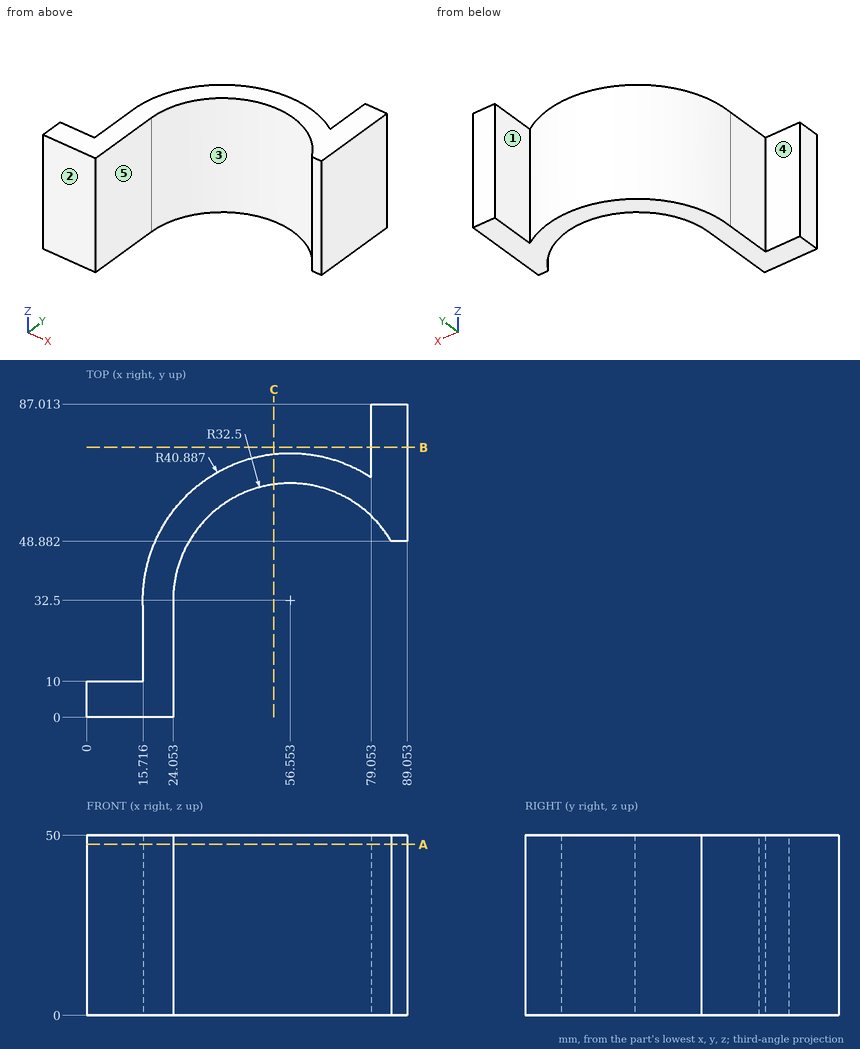
Can you work these out from the drawing? Everything is in mm from the part's minimum corner. A direction names the side the tool comes from. Coordinates: 2 decimals unless noted, no trailing zeros. Loops run counter-clockwise (first coordinate to the right, second up) from the corner with the lowest first, then second, coordinate; pieces in that order, holes last.
1) Imagine slicing it at A-A on z = 47.5. List the corners of the cut face in (x, y) for me.
2) Which directions (+Z, -Z, +X, -X, +Y, -Y) give clear straight access to the entire face, cutting with the end or side of a thin tool? Please do the marked faces 1 and 2.
3) For pin 1 (8 mm diameter, centred on x = 6.5, z = 18.5, fed in from +Y); pin 2 (16.5 mm diameter, centred on y = 19.5, z = 31.5, fed in from -X); pin 3 (3 mm diameter, centred on y = 31.5, z = 17, fed in from +X), each with a flat end and sliding along its axis, tell me the tip position at first contact or that it passes through.
4) Thinking about a two-plate mould opening in X: for the marked faces 3, 4 and 5, which applies, pulls with the +X half, pulls with the -X half, needs draft (parallel to the pull), parting line crosses it, or undercut?
5) Imagine slicing it at B-B on y = 75. List the corners of the cut face in (x, z) for me.
6) I need wall thicknesses on probe 1 along X at (y, z) = (14.5, 19.5); probe 2 along Y at (x, z) = (56, 28.5) (1 decimal); probe 3 along X at (y, z) = (9, 4.5). Which ranges of each line are inside material? Lowest first, please.
7) Imagine slicing it at C-C on x = 52. List the corners of the cut face in (y, z) for me.
Completed:
1. outline: (0, 0) - (24.05, 0) - (24.05, 32.5) arc R32.5 cw to (84.62, 48.88) - (89.05, 48.88) - (89.05, 87.01) - (79.05, 87.01) - (79.05, 66.64) arc R40.89 ccw to (15.72, 30.49) - (15.72, 10) - (0, 10) - close
2. face 1: +Z, -Z, +Y
2. face 2: +Z, -Z, +X, -X, -Y
3. pin 1: stops at y = 10
3. pin 2: stops at x = 15.72
3. pin 3: stops at x = 24.06
4. face 3: undercut
4. face 4: needs draft
4. face 5: pulls with the +X half
5. outline: (79.05, 0) - (89.05, 0) - (89.05, 50) - (79.05, 50) - close
6. probe 1: x = 15.72 to 24.05
6. probe 2: y = 65 to 73.4
6. probe 3: x = 0 to 24.05
7. outline: (64.68, 0) - (73.13, 0) - (73.13, 50) - (64.68, 50) - close
